Geometry check sheet. Reference: drawing and pictorial views, mm from the part's lowest x, y, z. Give positions to 0.01 mm unless a question says otherwise; leave off trailing zeros. Loops run counter-clockwise (first coordinate to the right, second up) from the corner with the lowest first, then second, coordinate; pieces in that order, holes last. Notation, with made-up numbers: (1.25, -26.5) -> (30.25, -26.5) arc R34 cw to (30.25, 8.5) -> close; hole circle Ø5 at (-37, 77). An arc over 180 degrees is marked (long way). Write each question's results on one line, items separated by ' | '. Start each with the question number.
1. Cross-section at B-B on z = 37. Record the boundary of the cut face in (x, y), and give its area (3 significant figures).
2. Material ranges on L1, parallel to Z at x = 37, y = 0.6; L2, parallel to Z at x = 37, y = 3.05, recorded low to high. Write a range as from..to.
3. Cross-section at C-C on z = 20.43. Record the boundary of the cut face in (x, y).
4. Mould release check, pull along X, two halves, no side actions. Record for the marked faces 1, 2 and 3: +X half, -X half, draft (parallel to the pull), parting line (faces both ways), or undercut.
5. Cross-section at A-A on x = 37. Record the boundary of the cut face in (y, z).
6. Cross-section at D-D on x = 26.5. Record the boundary of the cut face in (y, z).
7. Gauge pin test, flat ends, axial feed: pin 1 Ø9 at (x, z) = (51.35, 45.28) entering from -Y; pin 2 Ø1.5 at (x, y) = (54.5, 4.5) entering from -Z; pin 3 Ø2 at (y, z) = (2.5, 44) entering from -X; pin 4 Ø1.5 at (x, z) = (18, 45) entering from +Y. Record the tip position at first contact, or that the pin passes through.
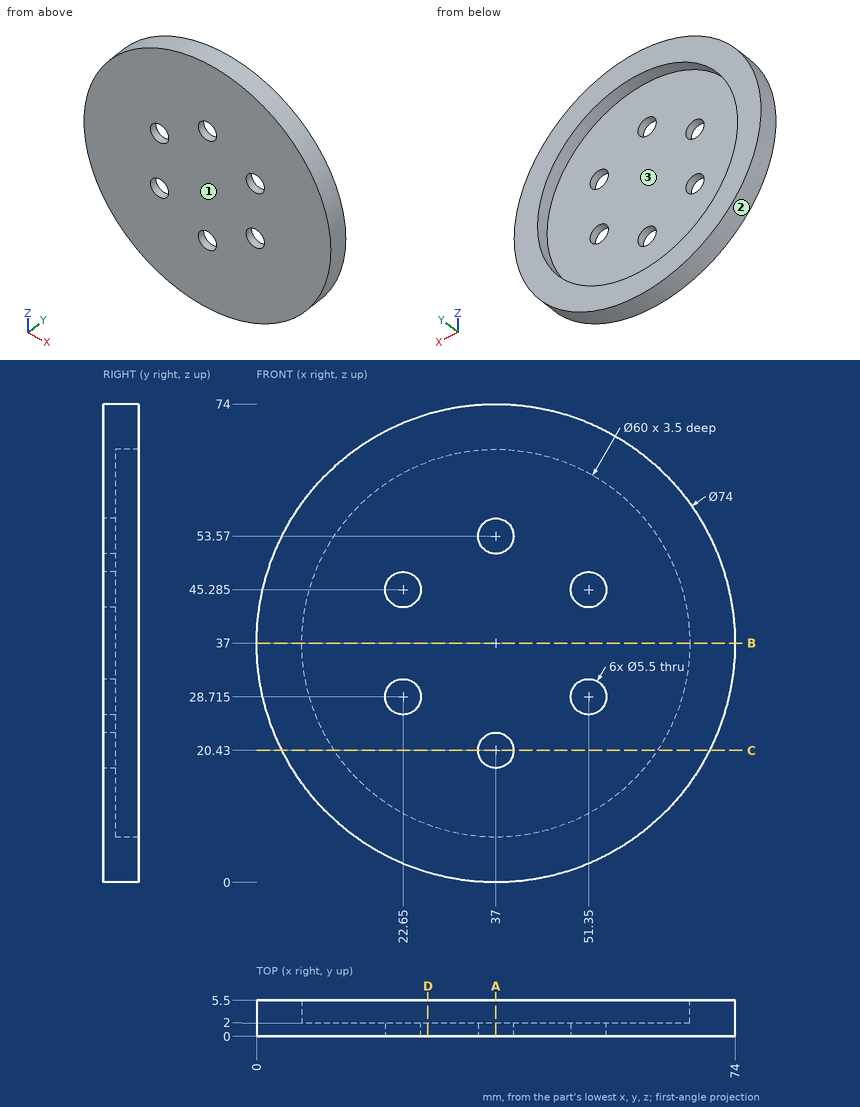
Geometry says:
1) outline: (0, 0) -> (74, 0) -> (74, 5.5) -> (67, 5.5) -> (67, 2) -> (7, 2) -> (7, 5.5) -> (0, 5.5) -> close | area: 197 mm^2
2) L1: 0..17.68, 23.18..50.82, 56.32..74 | L2: 0..7, 67..74
3) outline: (3.92, 0) -> (34.25, 0) -> (34.25, 2) -> (11.99, 2) -> (11.99, 5.5) -> (3.92, 5.5) -> close; (39.75, 0) -> (70.08, 0) -> (70.08, 5.5) -> (62.01, 5.5) -> (62.01, 2) -> (39.75, 2) -> close
4) face 1: draft | face 2: parting line | face 3: undercut
5) outline: (0, 0) -> (5.5, 0) -> (5.5, 7) -> (2, 7) -> (2, 17.68) -> (0, 17.68) -> close; (0, 23.18) -> (2, 23.18) -> (2, 50.82) -> (0, 50.82) -> close; (0, 56.32) -> (2, 56.32) -> (2, 67) -> (5.5, 67) -> (5.5, 74) -> (0, 74) -> close
6) outline: (0, 1.52) -> (5.5, 1.52) -> (5.5, 8.9) -> (2, 8.9) -> (2, 65.1) -> (5.5, 65.1) -> (5.5, 72.48) -> (0, 72.48) -> close
7) pin 1: y = 0 | pin 2: z = 4.01 | pin 3: x = 0.49 | pin 4: y = 2
